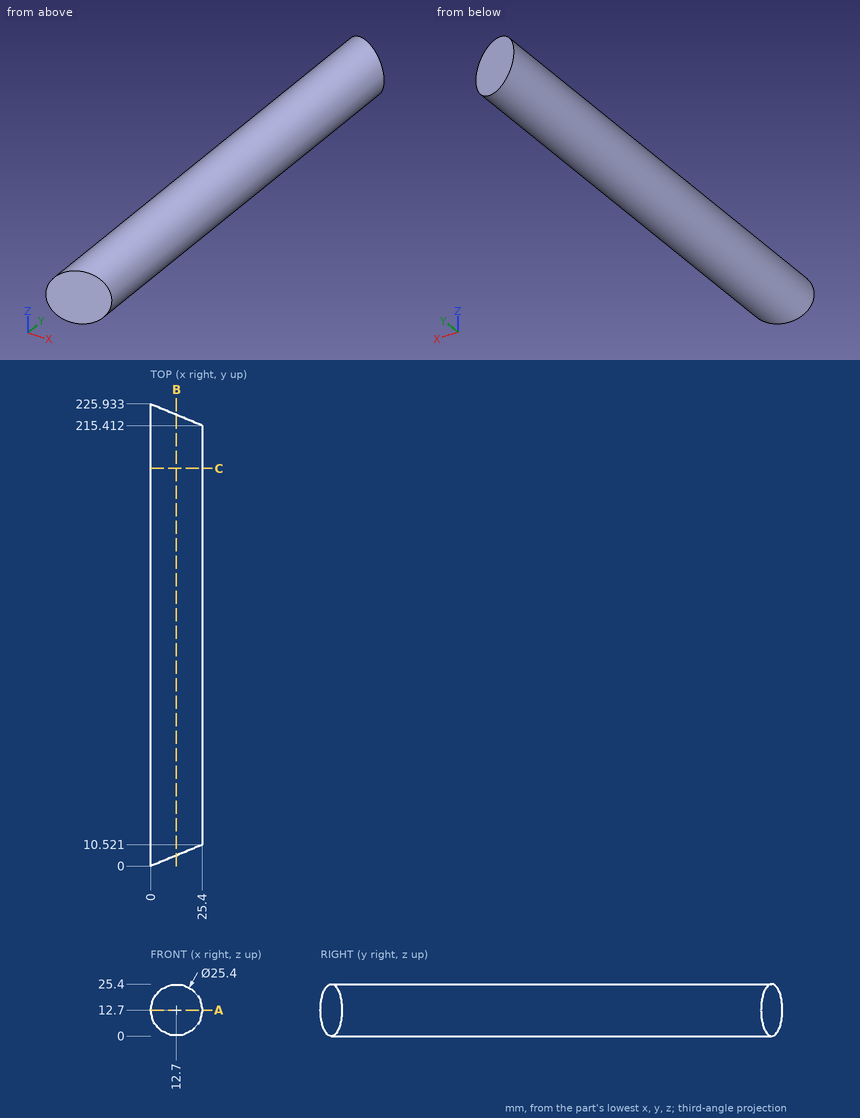
Drawing for the job (mm, zero at the part's lowest x, y, z). Give positions to 0.01 mm unless a question says otherwise; leave off trailing zeros. Order: outer loops, then holes, each group sorted by start corner. A loop starts at its lowest first (then second) coordinate and runs counter-clockwise, first axis right, second up. Notation, with made-up numbers: M -33,25 L 16,25 A15 cw 16,45 Z; hole C 10.25,42 d8. An arc over 180 degrees is marked long. Put each result on its own line as item: value. Start each with the question number.
(1) Saw through at B-B, the plane x = 12.7. Write the cut outline in (y, z).
(2) Drill centre lines: line 1 along Z through (x, y) = (12.25, 137); line 2 along Z through (x, y) = (10, 150); line 3 along X through (y, z) = (109, 14.25) (3 decimals). Where is each one in solid material? Low to high.
(3) Flat gauge pins, fed straight in: pin 1 Ø4 at (x, y) = (8.5, 162) entering from +Z; pin 2 Ø8 at (x, z) = (4.5, 8) entering from -Y; pin 3 Ø5 at (x, z) = (19.5, 22.5) entering from +Y. Where does each tip first touch, or does it go through?
(4) Saw through at C-C, the plane y = 194.5. Write the cut outline in (x, z).
(5) Saw through at A-A, the plane z = 12.7. Write the cut outline in (x, y), then the cut area to 3 significant figures.
Check result:
1. outline: M 5.26,0 L 220.67,0 L 220.67,25.4 L 5.26,25.4 Z
2. line 1: z = 0.01 to 25.39
2. line 2: z = 0.29 to 25.11
2. line 3: x = 0.095 to 25.305
3. pin 1: stops at z = 25.21
3. pin 2: stops at y = 0.25
3. pin 3: stops at y = 218.89
4. outline: C 12.7,12.7 d25.4
5. outline: M 0,0 L 25.4,10.52 L 25.4,215.41 L 0,225.93 Z
5. area: 5,470 mm2
